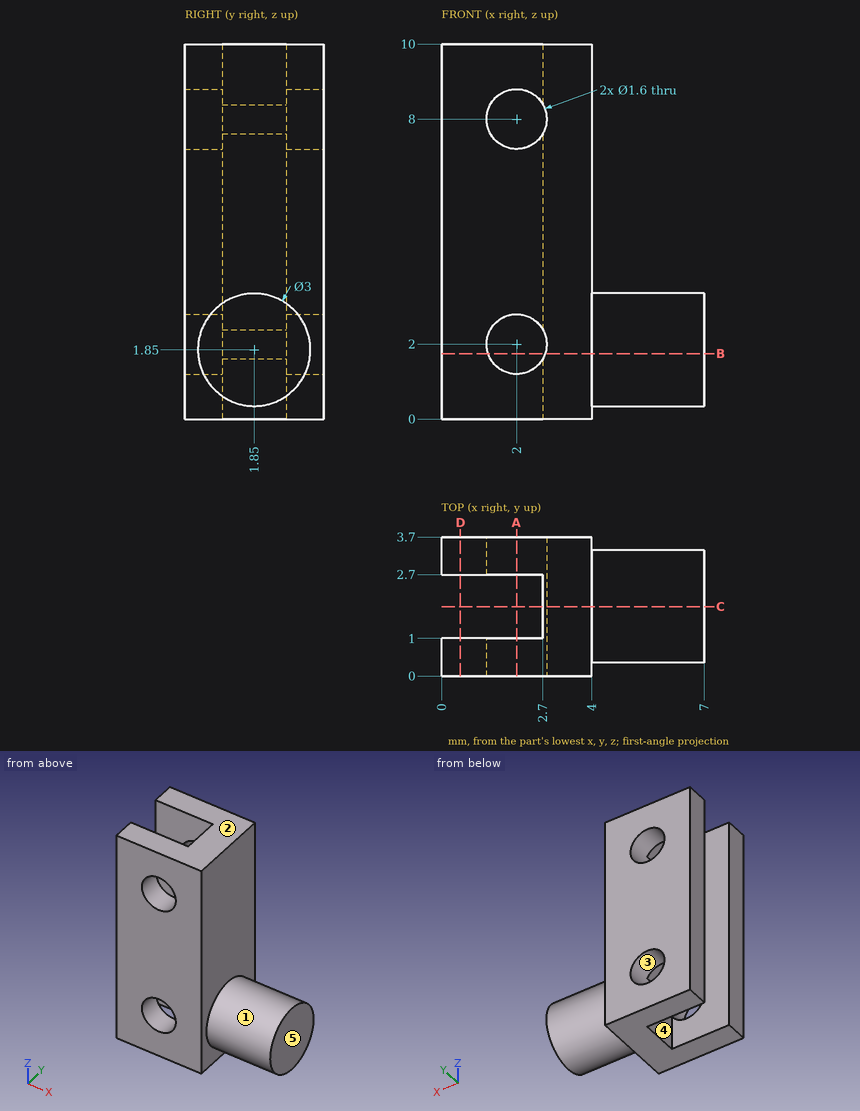
Here's the drawing with two shaded views (mm, measured from the low corner). I have some questions. A direction names the side the tool comes from. Round coordinates to 2 decimals unless told otherwise and drop trailing zeros. Loops run counter-clockwise (first coordinate to the right, second up) from the corner with the lowest first, then second, coordinate; pieces in that order, holes last. Notation, with made-up numbers: M 82.25,-2 L 137.25,-2 A15 cw 137.25,16 Z; hole C 24.5,-1 d11. An arc over 180 degrees is marked long. Answer as a JSON object with one key per item and string values. Group by question number.
Q1. Imagine slicing it at B-B, the plane z = 1.75. Please give me the cut outline in (x, y).
Q2. Will these pins go through, and if not, where does the flat tip stop? pin 1 (0.5 mm diameter, centred on y = 2, z = 5, fed in from -X); pin 2 (1 mm diameter, centred on y = 3, z = 7.5, fed in from +X).
Q3. Imagine slicing it at A-A, the plane x = 2. Please give me the cut outline in (y, z), then the cut area to 3 significant figures.
Q4. Imagine slicing it at D-D, the plane x = 0.5. Please give me the cut outline in (y, z), then the cut area to 3 significant figures.
Q5. We'd pull the mould along Z, two halves only. Please class the marked faces 1, 2 and 3: +Z half, -Z half, draft (parallel to the pull), parting line (faces both ways), or undercut.
Q6. Please list where these lines run through material, in increasing order: L1, parallel to Z at x = 2, y = 0.95; L2, parallel to Z at x = 1.5, y = 3.4; L3, parallel to X at y = 3.45, z = 2.
Q7. On a 3-axis mill with a long thin cutter (end or side, diameter ignored), from which of +Z, -Z, +X, -X, +Y, -Y can I reach the whole of each face in a straight line? I mean the marked faces 4 and 5. Say none if no direction works.
Q8. Imagine slicing it at C-C, the plane y = 1.85. Please give me the cut outline in (x, z).
Findings:
{
 "1": {"outline": "M 0,0 L 1.24,0 L 1.24,1 L 0,1 Z; M 0,2.7 L 1.24,2.7 L 1.24,3.7 L 0,3.7 Z; M 2.76,0 L 4,0 L 4,0.35 L 7,0.35 L 7,3.35 L 4,3.35 L 4,3.7 L 2.76,3.7 Z"},
 "2": {"pin 1": "stops at x = 2.7", "pin 2": "stops at x = 4"},
 "3": {"outline": "M 0,0 L 1,0 L 1,1.2 L 0,1.2 Z; M 0,2.8 L 1,2.8 L 1,7.2 L 0,7.2 Z; M 0,8.8 L 1,8.8 L 1,10 L 0,10 Z; M 2.7,0 L 3.7,0 L 3.7,1.2 L 2.7,1.2 Z; M 2.7,2.8 L 3.7,2.8 L 3.7,7.2 L 2.7,7.2 Z; M 2.7,8.8 L 3.7,8.8 L 3.7,10 L 2.7,10 Z", "area": "13.6 mm2"},
 "4": {"outline": "M 0,0 L 1,0 L 1,10 L 0,10 Z; M 2.7,0 L 3.7,0 L 3.7,10 L 2.7,10 Z", "area": "20.0 mm2"},
 "5": {"face 1": "parting line", "face 2": "+Z half", "face 3": "undercut"},
 "6": {"L1": "z = 0 to 1.2, 2.8 to 7.2, 8.8 to 10", "L2": "z = 0 to 1.38, 2.62 to 7.38, 8.62 to 10", "L3": "x = 0 to 1.2, 2.8 to 4"},
 "7": {"face 4": "+Z, -Z, -X", "face 5": "+Z, -Z, +X, +Y, -Y"},
 "8": {"outline": "M 2.7,0 L 4,0 L 4,0.35 L 7,0.35 L 7,3.35 L 4,3.35 L 4,10 L 2.7,10 L 2.7,8.39 A0.8 cw 2.7,7.61 L 2.7,2.39 A0.8 cw 2.7,1.61 Z"}
}
